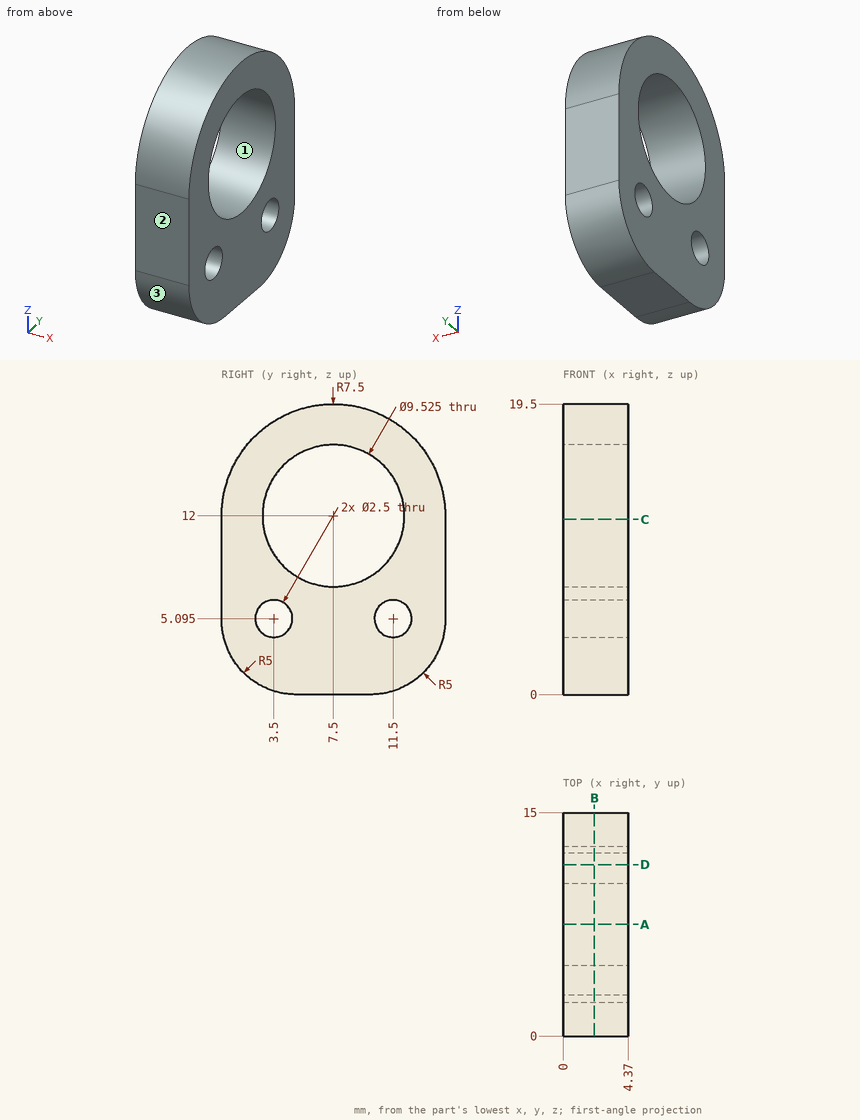
Can you work these out from the drawing? Everything is in mm from the part's minimum corner. Coordinates: 2 decimals unless noted, no trailing zeros. Loops run counter-clockwise (first coordinate to the right, second up) from the corner with the lowest first, then second, coordinate; pieces in that order, holes last.
1) Thinking about a two-plate mould opening in Z: for the marked faces 1, 2 and 3, which applies, pulls with the +Z half, pulls with the -Z half, needs draft (parallel to the pull), parting line crosses it, or undercut?
2) Imagine slicing it at B-B on x = 2.1. State how many separate pieces and enclosed holes the cut face has, plus the area to 3 significant figures.
3) Imagine slicing it at D-D on y = 11.5. List the corners of the cut face in (x, z) for me (1 decimal).
4) I need wall thicknesses on probe 1 along Z at (x, y) = (1.55, 10.5) (1 decimal); probe 2 along Z at (x, y) = (3.05, 4.25) (1 decimal); probe 3 along Y at (x, z) = (2.1, 4.25). Which ranges of each line are inside material? Lowest first, please.
5) Imagine slicing it at A-A on y = 7.5. List the corners of the cut face in (x, z) for me, plus the area to 3 significant figures.
6) Imagine slicing it at C-C on z = 11.75. List the corners of the cut face in (x, y) for me.
Completed:
1. face 1: undercut
1. face 2: needs draft
1. face 3: pulls with the -Z half
2. separate pieces: 1
2. enclosed holes: 3
2. area: 177 mm2
3. outline: (0, 0.2) - (4.4, 0.2) - (4.4, 3.8) - (0, 3.8) - close; (0, 6.3) - (4.4, 6.3) - (4.4, 9.4) - (0, 9.4) - close; (0, 14.6) - (4.4, 14.6) - (4.4, 18.3) - (0, 18.3) - close
4. probe 1: z = 0 to 4.3, 5.8 to 8.3, 15.7 to 18.9
4. probe 2: z = 0.1 to 4.1, 6.1 to 8.5, 15.5 to 18.8
4. probe 3: y = 0.06 to 2.58, 4.42 to 10.58, 12.42 to 14.94
5. outline: (0, 0) - (4.37, 0) - (4.37, 7.24) - (0, 7.24) - close; (0, 16.76) - (4.37, 16.76) - (4.37, 19.5) - (0, 19.5) - close
5. area: 43.6 mm2
6. outline: (0, 0) - (4.37, 0) - (4.37, 2.74) - (0, 2.74) - close; (0, 12.26) - (4.37, 12.26) - (4.37, 15) - (0, 15) - close
